Read the model definition and answer for the solid it produces. Units are mm, in the model's axes. Face numbers are marked on the shaded views. A direction names the side the tool comes from. Coordinates: 2 decimals unless noted, no trailing zeros. Loops run counter-clockwise (first coordinate to the right, second up) from the corner with the lowest first, then second, coordinate; pieces in that order, holes last. Notation, with made-up numbers: (16, -33) - (68, -33) arc R30 ccw to (68, -4) - close; hole circle Ø11 at (-25, 55). An arc over 180 degrees is marked (long way). Use one line per item in the form item = value.
from build123d import *

# Parameters (mm, degrees)
F1_DEPTH = 50
F4_DEPTH = 47
F5_R     = 26
F6_DEPTH = 15
F8_W     = 2
F8_H     = 13.5


with BuildPart() as f1:
    # F0 (on Front) → F1 (new body)
    with BuildSketch(Plane.XZ):
        with BuildLine():
            ThreePointArc((56.5, 50.8306010195), (30.9263182623, 69.4230713721), (0, 76))
            ThreePointArc((0, 76), (-75.8948480637, 3.9965031459), (-7.9819473433, -75.5796832264))
            Line((-7.9819473433, -75.5796832264), (8.4910760519, -75.5241790917))
            ThreePointArc((8.4910760519, -75.5241790917), (34.7620941702, -67.5839981719), (56.5, -50.8306010195))
            ThreePointArc((56.5, -50.8306010195), (37, 0), (56.5, 50.8306010195))
        make_face()
        with BuildLine():
            Line((113, 76), (0, 76))
            ThreePointArc((0, 76), (30.9263182623, 69.4230713721), (56.5, 50.8306010195))
            ThreePointArc((56.5, 50.8306010195), (82.0736817377, 69.4230713721), (113, 76))
        make_face()
        with BuildLine():
            ThreePointArc((113, 76), (82.0736817377, 69.4230713721), (56.5, 50.8306010195))
            ThreePointArc((56.5, 50.8306010195), (76, 0), (56.5, -50.8306010195))
            ThreePointArc((56.5, -50.8306010195), (77.1458775127, -67.0110580477), (102.0628366951, -75.2088988009))
            Line((102.0628366951, -75.2088988009), (124.4437263036, -75.133488727))
            ThreePointArc((124.4437263036, -75.133488727), (188.7830625643, 5.7382426207), (113, 76))
        make_face()
        with BuildLine():
            ThreePointArc((56.5, -50.8306010195), (76, 0), (56.5, 50.8306010195))
            ThreePointArc((56.5, 50.8306010195), (37, 0), (56.5, -50.8306010195))
        make_face()
        with BuildLine():
            ThreePointArc((56.5, -50.8306010195), (34.7620941702, -67.5839981719), (8.4910760519, -75.5241790917))
            Line((8.4910760519, -75.5241790917), (102.0628366951, -75.2088988009))
            ThreePointArc((102.0628366951, -75.2088988009), (77.1458775127, -67.0110580477), (56.5, -50.8306010195))
        make_face()
    extrude(amount=F1_DEPTH)

    # F3 (on offset) → F4 (cut)
    with BuildSketch(Plane.XZ.offset(19)):
        with BuildLine():
            Line((-10.5, -61.611687203), (-10.5, 61.611687203))
            ThreePointArc((-10.5, 61.611687203), (-62.5, 0), (-10.5, -61.611687203))
        make_face()
        Polygon((128.5, 60.5475020129), (-10.5, 61.611687203), (-10.5, -61.611687203), (128.5, -60.5475020129), align=None)
        with BuildLine():
            ThreePointArc((128.5, -60.5475020129), (175.5, 0), (128.5, 60.5475020129))
            Line((128.5, 60.5475020129), (128.5, -60.5475020129))
        make_face()
    extrude(amount=F4_DEPTH, mode=Mode.SUBTRACT)

    # F5 (on offset) → F6 (cut)
    with BuildSketch(Plane.XZ.offset(19)):
        Circle(F5_R)
    extrude(amount=-F6_DEPTH, mode=Mode.SUBTRACT)

    # F8 (on offset) → F9 (revolve, cut)
    with BuildSketch(Plane.YZ.offset(111)):
        with Locations((-1, 6.75)):
            Rectangle(F8_W, F8_H)
        Polygon((-17, 0), (-2, 0), (-2, 13.5), (-2, 18.5), (-7, 18.5), (-7, 23.5), (-19, 23.5), (-19, 0), align=None)
    revolve(axis=Axis((111, -8.5, 0), (0, 1, 0)), mode=Mode.SUBTRACT)


solid = f1.part
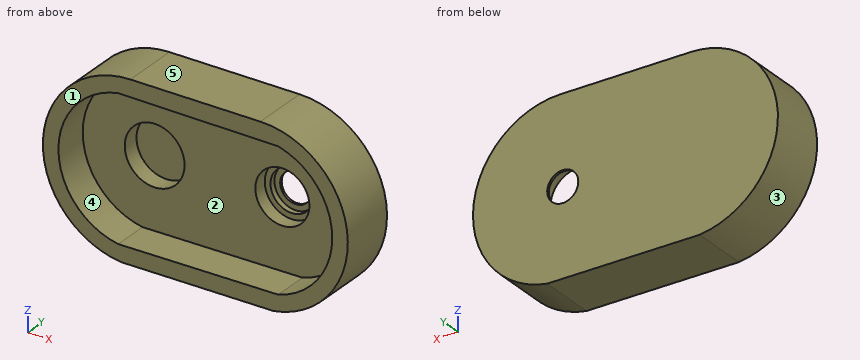
Item 1: The part is cut by section C-C on x = 118.5. Give the vertices of the cut face in (y, z), plus the area to 3 significant figures.
Results below:
outline = (-50, -75.15) - (0, -75.15) - (0, -11.22) - (-2, -11.22) - (-2, -16.91) - (-7, -16.91) - (-7, -22.27) - (-19, -22.27) - (-19, -60.62) - (-50, -60.62) - close; (-50, 60.62) - (-19, 60.62) - (-19, 22.27) - (-7, 22.27) - (-7, 16.91) - (-2, 16.91) - (-2, 11.22) - (0, 11.22) - (0, 75.8) - (-50, 75.8) - close
area = 3,040 mm²
Item 2: The part is cut by section A-A on z = 0. Give the vertices of the cut face in (x, y), plus the area to 3 significant figures.
Results below:
outline = (-76, -50) - (-62.5, -50) - (-62.5, -19) - (-26, -19) - (-26, -4) - (26, -4) - (26, -19) - (87.5, -19) - (87.5, -7) - (92.5, -7) - (92.5, -2) - (97.5, -2) - (97.5, 0) - (-76, 0) - close; (124.5, -2) - (129.5, -2) - (129.5, -7) - (134.5, -7) - (134.5, -19) - (175.5, -19) - (175.5, -50) - (189, -50) - (189, 0) - (124.5, 0) - close
area = 4,290 mm²
Item 3: For a pull along Z with two mould halves and no side action, classify the marked faces 1, 2 and 3 as +Z half, -Z half, draft (parallel to the pull), parting line (faces both ways), or undercut.
Results below:
face_1 = draft
face_2 = undercut
face_3 = parting line
Item 4: Find the intervals of material crossed by L1, parallel to Z at x = 0, y = -10; L2, parallel to Y at x = 126.5, z = -27; L3, parallel to X at y = -1.3, z = 0, in increasing order.
Results below:
L1 = -75.55 to -26, 26 to 76
L2 = -19 to 0
L3 = -76 to 97.5, 124.5 to 189
Item 5: Which of the six approach directions +Z, -Z, +X, -X, +Y, -Y give full straight-line access (tool end or side, diameter ignored) to the marked faces 4 and 5?
Results below:
face_4 = -Y
face_5 = +Z, +X, -X, +Y, -Y
Item 6: The part is cut by section B-B on y = -37.5. Give the vertices of the cut face in (x, z).
Results below:
outline = (-7.98, -75.58) - (124.44, -75.13) arc R76 ccw to (113, 76) - (0, 76) arc R76 ccw to start; hole (-10.5, -61.61) - (128.5, -60.55) arc R62.5 ccw to (128.5, 60.55) - (-10.5, 61.61) arc R62.5 ccw to start
Item 7: Each of these flat-tipped pins is pushed along its axis until it touches: P1, Ø15.5, axis at x = 0.5, z = -2.5, coming from the -Y side; P2, Ø18.5, axis at x = 106.5, z = 2.5, coming from the -Y side; P3, Ø2, axis at x = 27, z = 7.5, coming from the -Y side. Where does it stop, or does it pass through?
Results below:
P1 = -4
P2 = -2
P3 = -19
Item 8: The part is cut by section D-D on x = 59. Give the vertices of the cut face in (y, z), plus the area to 3 significant figures.
Results below:
outline = (-50, -75.35) - (0, -75.35) - (0, 76) - (-50, 76) - (-50, 61.08) - (-19, 61.08) - (-19, -61.08) - (-50, -61.08) - close
area = 3,780 mm²
